```python
from build123d import *

# Parameters (mm, degrees)
F0_W      = 35.84
F0_H      = 7.07
F1_DEPTH  = 45
F4_W      = 6.89
F4_H      = 40.5
F5_DEPTH  = 7.07
F6_W      = 6.89
F6_H      = 40.5
F7_DEPTH  = 7.07
F2_W      = 14
F2_H      = 7.07
F9_DEPTH  = 7.6
F10_W     = 13.65
F10_H     = 23.4
F11_DEPTH = 7.07
F12_W     = 13.65
F12_H     = 5
F13_DEPTH = 2.6
F14_W     = 13.825
F14_H     = 5.35
F15_DEPTH = 2.8
F16_R     = 3
F17_R     = 1.25
F18_DEPTH = 4.27
F19_R     = 1.25
F20_DEPTH = 4.47


with BuildPart() as f1:
    # F0 (on Top) → F1 (new body)
    with BuildSketch(Plane.XY):
        Rectangle(F0_W, F0_H)
    extrude(amount=F1_DEPTH)

    # F4 (on face) → F5 (cut, through all)
    with BuildSketch(Plane.XZ.offset(3.535)):
        with Locations((14.475, 24.75)):
            Rectangle(F4_W, F4_H)
    extrude(amount=-F5_DEPTH, mode=Mode.SUBTRACT)

    # F6 (on face) → F7 (cut, through all)
    with BuildSketch(Plane.XZ.offset(3.535)):
        with Locations((-14.475, 24.75)):
            Rectangle(F6_W, F6_H)
    extrude(amount=-F7_DEPTH, mode=Mode.SUBTRACT)

    # F2 (on face) → F9 (cut)
    with BuildSketch(Plane(origin=(0, 0, 0), x_dir=(1, 0, 0), z_dir=(0, 0, -1))):
        Rectangle(F2_W, F2_H)
    extrude(amount=-F9_DEPTH, mode=Mode.SUBTRACT)

    # F10 (on face) → F11 (cut, through all)
    with BuildSketch(Plane(origin=(0, 3.535, 0), x_dir=(-1, 0, 0), z_dir=(0, 1, 0))):
        with Locations((0, 24.65)):
            Rectangle(F10_W, F10_H)
    extrude(amount=-F11_DEPTH, mode=Mode.SUBTRACT)

    # F12 (on face) → F13 (cut)
    with BuildSketch(Plane(origin=(0, 3.535, 0), x_dir=(-1, 0, 0), z_dir=(0, 1, 0))):
        with Locations((0, 38.85)):
            Rectangle(F12_W, F12_H)
    extrude(amount=-F13_DEPTH, mode=Mode.SUBTRACT)

    # F14 (on face) → F15 (cut)
    with BuildSketch(Plane(origin=(0, 3.535, 0), x_dir=(-1, 0, 0), z_dir=(0, 1, 0))):
        with Locations((0.0875, 10.275)):
            Rectangle(F14_W, F14_H)
    extrude(amount=-F15_DEPTH, mode=Mode.SUBTRACT)

    # F16
    f16_edges = [f1.edges().sort_by_distance(p)[0] for p in [
        (-11.03, 0, 4.5),
        (11.03, 0, 4.5),
    ]]
    fillet(f16_edges, radius=F16_R)

    # F17 (on face) → F18 (cut, through all)
    with BuildSketch(Plane(origin=(0, 0.735, 0), x_dir=(-1, 0, 0), z_dir=(0, 1, 0))):
        with Locations((0.04375, 10.275)):
            Circle(F17_R)
    extrude(amount=-F18_DEPTH, mode=Mode.SUBTRACT)

    # F19 (on face) → F20 (cut, through all)
    with BuildSketch(Plane(origin=(0, 0.935, 0), x_dir=(-1, 0, 0), z_dir=(0, 1, 0))):
        with Locations((0, 38.85)):
            Circle(F19_R)
    extrude(amount=-F20_DEPTH, mode=Mode.SUBTRACT)


solid = f1.part
```
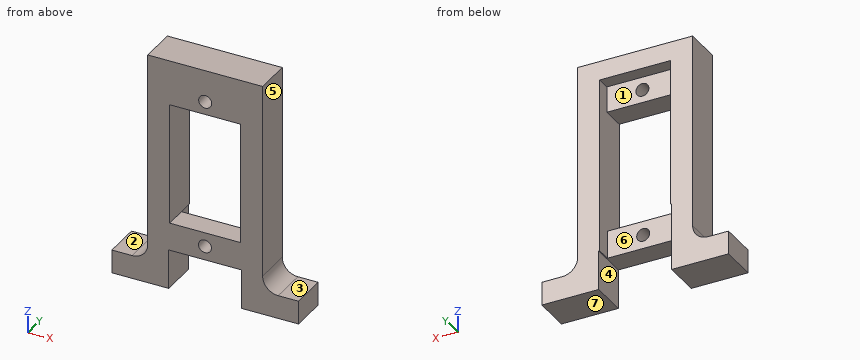
CAD build for the part. Positions are in the model's coordinates, mm. Face numbers are marked on the shaded views. A direction names the side the tool comes from. Round coordinates to 2 decimals unless told otherwise and drop trailing zeros. Write each loop counter-clockwise with the first axis right and the second up, starting at its lowest first coordinate (ties: lowest second). Pieces come first, ordered by that corner, then holes. Notation, with made-up numbers: (10, 1) - (36, 1) arc R10 cw to (36, 15) - close; hole circle Ø5 at (-21, 21.25). An arc over 180 degrees is marked (long way). Return JSON: item names as keys, results as strings. Group by question number.
Item 1: 3-axis set-ups, long thin cutter, end or side, ignore diameter. For the marked faces 1, 2, 3 and 4: which of +Z, -Z, +X, -X, +Y, -Y reach the whole face in a straight line?
Item 2: Mould opens along X. For the marked faces 5, 6 and 7 say: +X half, -X half, draft (parallel to the pull), parting line (faces both ways), or undercut.
Item 3: Band-saw the part on D-D on z = 26. List the corners of the cut face in (x, y) (3 decimals), plus the area to 3 significant figures.
Item 4: Flat gauge pins, fed straight in: pin 1 Ø2 at (x, y) = (2, 3) entering from -Z; pin 2 Ø1.6 at (x, z) = (-3, 11.5) entering from +Y (3 decimals); pin 3 Ø3.5 at (x, y) = (2.5, -1) entering from -Z. Where does each tip first touch, or does it go through?
Item 5: Band-saw the part on A-A on z = 38.85. List the corners of the cut face in (x, y) (3 decimals).
Item 6: Band-saw the part on B-B on x = -4. List the corners of the cut face in (y, z) (3 decimals), plus the area to 3 significant figures.
Item 7: Band-saw the part on C-C on y = 0. List the corners of the cut face in (x, z) (3 decimals), plus the area to 3 significant figures.
Item 8: Probe probe 1 along Z at (x, y) = (0, -2.15); probe 2 along X at (y, z) = (-1, 14.5) (3 decimals). List the from-to ranges inside material, lowest first.
Resolved:
{
 "1": {"face 1": "-Z, +Y", "face 2": "+Z, -X, +Y, -Y", "face 3": "+Z, +X, +Y, -Y", "face 4": "-Z, +Y, -Y"},
 "2": {"face 5": "+X half", "face 6": "undercut", "face 7": "draft"},
 "3": {"outline": "(-11.03, -3.535) - (-6.825, -3.535) - (-6.825, 3.535) - (-11.03, 3.535) - close; (6.825, -3.535) - (11.03, -3.535) - (11.03, 3.535) - (6.825, 3.535) - close", "area": "59.5 mm²"},
 "4": {"pin 1": "stops at z = 41.35", "pin 2": "stops at y = 0.735", "pin 3": "stops at z = 7.6"},
 "5": {"outline": "(-11.03, -3.535) - (-1.25, -3.535) - (-1.25, 0.935) - (-6.825, 0.935) - (-6.825, 3.535) - (-11.03, 3.535) - close; (1.25, -3.535) - (11.03, -3.535) - (11.03, 3.535) - (6.825, 3.535) - (6.825, 0.935) - (1.25, 0.935) - close"},
 "6": {"outline": "(-3.535, 7.6) - (0.735, 7.6) - (0.735, 12.95) - (-3.535, 12.95) - close; (-3.535, 36.35) - (0.935, 36.35) - (0.935, 41.35) - (3.535, 41.35) - (3.535, 45) - (-3.535, 45) - close", "area": "71.0 mm²"},
 "7": {"outline": "(-17.92, 0) - (-7, 0) - (-7, 7.6) - (7, 7.6) - (7, 0) - (17.92, 0) - (17.92, 4.5) - (14.03, 4.5) arc R3 cw to (11.03, 7.5) - (11.03, 45) - (-11.03, 45) - (-11.03, 7.5) arc R3 cw to (-14.03, 4.5) - (-17.92, 4.5) - close; hole (-6.825, 12.95) - (6.825, 12.95) - (6.825, 36.35) - (-6.825, 36.35) - close; hole circle Ø2.5 at (-0.044, 10.275); hole circle Ø2.5 at (0, 38.85)", "area": "623 mm²"},
 "8": {"probe 1": "z = 7.6 to 9.03, 11.52 to 12.95, 36.35 to 37.6, 40.1 to 45", "probe 2": "x = -11.03 to -6.825, 6.825 to 11.03"}
}
